from build123d import *

# Parameters (mm, degrees)
SKETCH_1_W                  = 196
SKETCH_1_H                  = 118
EXTRUDE_1_DEPTH             = 17
HOLE_WIZARD_M31_D           = 3.242
HOLE_WIZARD_M31_DEPTH       = 11.218815752
HOLE_WIZARD_M31_TIP         = 0.935884786
HOLE_WIZARD_M81_D           = 9
HOLE_WIZARD_M81_CBORE_D     = 15
HOLE_WIZARD_M81_CBORE_DEPTH = 11
CHAMFER_1_SIZE              = 0.379


with BuildPart() as part:
    # Эскиз1 → Бобышка-Вытянуть1 (new body)
    with BuildSketch(Plane.XY.offset(17)):
        Rectangle(SKETCH_1_W, SKETCH_1_H)
    extrude(amount=-EXTRUDE_1_DEPTH)

    # Отверстие с зазором M31
    with Locations(Plane.XY.offset(17)):
        with Locations((-83, 48), (-83, -48), (83, 48), (83, -48)):
            Hole(HOLE_WIZARD_M31_D / 2, depth=HOLE_WIZARD_M31_DEPTH)
            with Locations((0, 0, -(HOLE_WIZARD_M31_DEPTH + HOLE_WIZARD_M31_TIP / 2))):  # 120° drill point
                Cone(0, HOLE_WIZARD_M31_D / 2, HOLE_WIZARD_M31_TIP, mode=Mode.SUBTRACT)

    # Цековка для  болта с шестигранной головкой M81 (through all)
    with Locations(Plane.XY.offset(17)):
        with Locations((66, 48), (66, -48), (-66, 48), (-66, -48)):
            CounterBoreHole(HOLE_WIZARD_M81_D / 2, HOLE_WIZARD_M81_CBORE_D / 2, HOLE_WIZARD_M81_CBORE_DEPTH)

    # Фаска1
    chamfer_1_edges = [part.edges().sort_by_distance(p)[0] for p in [
        (84.621, -48, 17),
        (84.621, 48, 17),
        (-81.379, -48, 17),
        (-81.379, 48, 17),
    ]]
    chamfer(chamfer_1_edges, length=CHAMFER_1_SIZE)


solid = part.part
Can you work these out from the model? Positions are in its coordinate system, mm. A direction names the side the tool comes from. Coordinates: 2 decimals unless noted, no trailing zeros. Write each loop counter-clockwise with the first axis right and the second up, starting at its lowest first coordinate (ties: lowest second). Pieces come first, ordered by that corner, then holes. Notation, with made-up numbers: M 17.25,30.25 L 21.25,30.25 A6 cw 21.25,40.25 Z; hole C 22,78 d7. An arc over 180 degrees is marked long. Use one line per item in the form item = value.
Q1. I need wall thicknesses on line 1 along X through (y, z) = (-42, 13); line 2 along Y through (x, z) = (66, 4.6); line 3 along Y through (x, z) = (83, 12.5). Which ranges of each line are inside material? Lowest first, please. Write a range as from..to.
Model answer:
line_1 = -98..-70.5, -61.5..61.5, 70.5..98
line_2 = -59..-52.5, -43.5..43.5, 52.5..59
line_3 = -59..-49.62, -46.38..46.38, 49.62..59
Q2. We'd pull the mould along X, two halves only. Please class faces 1 (the cylindrical face through (63.92, -51.99, 2.96)), 2 (the flat face through (-1, 59, 9)): +X half, -X half, draft (parallel to the pull), parting line (faces both ways), or undercut.
Model answer:
face_1 = undercut
face_2 = draft
Q3. For faces 3 (the flat face through (-66, 43, 6)), 4 (the cylindrical face through (63.92, 44.01, 2.96)), which set-ups out of +Z, -Z, +X, -X, +Y, -Y let a thin tool reach every point of the face, with its end or its side?
Model answer:
face_3 = +Z
face_4 = +Z, -Z
Q4. If we section it at B-B (z = 9): State how many separate pieces and enclosed holes the cut face has, then the cut area to 3 significant figures.
Model answer:
separate_pieces = 1
enclosed_holes = 8
area = 22,400 mm^2
Q5. For P1, Ø8, axis at x = -66, y = 48, coming from the +Z side; P2, Ø11.5, axis at x = -66, y = -48, coming from the +Z side; P3, Ø3, axis at x = -83, y = 48, coming from the +Z side; P4, Ø2.5, axis at x = 83, y = -48, coming from the +Z side, each with a flat end and sliding along its axis, tell me the tip position at first contact or that it passes through.
Model answer:
P1 = through
P2 = 6
P3 = 5.71
P4 = 5.57
Q6. If we section it at A-A (x = -66): Write out the boundary of the cut face in (y, z), then the cut area to 3 significant figures.
Model answer:
outline = M -59,0 L -52.5,0 L -52.5,6 L -55.5,6 L -55.5,17 L -59,17 Z; M -43.5,0 L 43.5,0 L 43.5,6 L 40.5,6 L 40.5,17 L -40.5,17 L -40.5,6 L -43.5,6 Z; M 52.5,0 L 59,0 L 59,17 L 55.5,17 L 55.5,6 L 52.5,6 Z
area = 1,570 mm^2
